from build123d import *

# Parameters (mm, degrees)
F0_R     = 12.5
F0_R_2   = 9.5
F1_DEPTH = 5
F2_R     = 0.9198153673


# Not quite as in the source:
# - a fillet or chamfer that OpenCascade refuses, or shapes differently, is made with other operations: its cross-section is extruded or revolved along the edge and cut away or added


with BuildPart() as f1:
    # F0 (on Top) → F1 (new body)
    with BuildSketch(Plane.XY):
        Circle(F0_R)
        Circle(F0_R_2, mode=Mode.SUBTRACT)
    extrude(amount=F1_DEPTH)

    # F2
    f2_edges = [f1.edges().sort_by_distance(p)[0] for p in [
        (-9.5, 0, 5),
        (-9.5, 0, 0),
    ]]
    fillet(f2_edges, radius=F2_R)

    # F3: fillet of radius 2.1462358569 on 2 edges, made by hand

    # F3_s1 → F3_t2 (revolve, cut)
    with BuildSketch(Plane.XZ):
        with BuildLine():
            ThreePointArc((10.4198153673, 0), (11.8945577469, 0.6511364368), (12.5, 2.1452192404))
            Line((12.5, 2.1452192404), (12.5429247171, 2.1452192404))
            Line((12.5429247171, 2.1452192404), (12.5429247171, 0))
            Line((12.5429247171, 0), (12.5, -0.0429247171))
            ThreePointArc((12.5, -0.0429247171), (11.4599076836, -0.0429247171), (10.4211363917, -0.0429043848))
            Line((10.4211363917, -0.0429043848), (10.4198153673, 0))
        make_face()
    revolve(axis=Axis((0, 0, 0), (0, 0, 1)), mode=Mode.SUBTRACT)

    # F3_s3 → F3_t4 (revolve, cut)
    with BuildSketch(Plane.XZ):
        with BuildLine():
            ThreePointArc((10.4198153673, 5), (11.8945577469, 4.3488635632), (12.5, 2.8547807596))
            Line((12.5, 2.8547807596), (12.5429247171, 2.8547807596))
            Line((12.5429247171, 2.8547807596), (12.5429247171, 5))
            Line((12.5429247171, 5), (12.5, 5.0429247171))
            ThreePointArc((12.5, 5.0429247171), (11.4599076836, 5.0429247171), (10.4211363917, 5.0429043848))
            Line((10.4211363917, 5.0429043848), (10.4198153673, 5))
        make_face()
    revolve(axis=Axis((0, 0, 5), (0, 0, 1)), mode=Mode.SUBTRACT)


solid = f1.part
Model file for the job. Use its own axes, mm. Round coordinates to 2 decimals unless told otherwise and drop trailing zeros. Order: outer loops, then holes, each group sorted by start corner. A loop starts at its lowest first (then second) coordinate and runs counter-clockwise, first axis right, second up.
(1) Band-saw the part on C-C (z = 2.5). List the corners of the cut face in (x, y), then the cut area to 3 significant figures.
(2) Pull direction Y, two halves, no side cores. Call faces 1 (the face through (11.923, 3.755, 2.495)), 2 (the face through (4.38, -8.43, 2.48)): released by +Y, released by -Y, zero draft, split by the parting line, or undercut.
(3) Band-saw the part on A-A (y = 0). List the corners of the cut face in (x, z).
(4) Drill centre lines: line 1 (Y direction, x = 0, z = 2.35); line 2 (Y direction, x = 3.75, z = 3.95); line 3 (X direction, y = 7.5, z = 4.4). Where is each one in solid material? Low to high.
(5) Pin check, flat tips, straight feed: pin 1 (3 mm diameter, centred on y = -9.5, z = 1.5, fed in from -X); pin 2 (2 mm diameter, centred on y = 5, z = 2, fed in from +X); pin 3 (1 mm diameter, centred on y = -4, z = 1.5, fed in from +X). Stop position of each tip, or through.
Verdict:
1. outline: circle Ø25 at (0, 0); hole circle Ø19 at (0, 0)
1. area: 207 mm2
2. face 1: split by the parting line
2. face 2: undercut
3. outline: (-12.5, 2.15) arc R2.15 ccw to (-10.42, 0) arc R0.92 ccw to (-9.5, 0.92) - (-9.5, 4.08) arc R0.92 ccw to (-10.42, 5) arc R2.15 ccw to (-12.5, 2.85) - close; (9.5, 0.92) arc R0.92 ccw to (10.42, 0) arc R2.15 ccw to (12.5, 2.15) - (12.5, 2.85) arc R2.15 ccw to (10.42, 5) arc R0.92 ccw to (9.5, 4.08) - close
4. line 1: y = -12.5 to -9.5, 9.5 to 12.5
4. line 2: y = -11.61 to -8.73, 8.73 to 11.61
4. line 3: x = -9.17 to -5.92, 5.92 to 9.17
5. pin 1: stops at x = -9.54
5. pin 2: stops at x = 11.84
5. pin 3: stops at x = 11.94
